```python
from build123d import *

# Parameters (mm, degrees)
F0_R            = 7.62
F1_DEPTH        = 25.4
F2_SIZE         = 2.54
F4_DEPTH        = 25.4
F4_COPIES_COUNT = 18
F6_R            = 5.08
F7_DEPTH        = 12.954
F8_R            = 5.08
F9_DEPTH        = 12.7


# Not quite as in the source:
# - a pattern or mirror of a feature is missing from the dataset's text; its kind, count and spacing are read off the source's solid


with BuildPart() as f1:
    # F0 (on Top) → F1 (new body)
    with BuildSketch(Plane.XY):
        Circle(F0_R)
    extrude(amount=F1_DEPTH)

    # F2
    f2_edges = [f1.edges().sort_by_distance(p)[0] for p in [
        (-7.62, 0, 25.4),
        (-7.62, 0, 0),
    ]]
    chamfer(f2_edges, length=F2_SIZE)

    # F3 (on face) → F4 (cut, through all)
    with BuildSketch(Plane.XY.offset(25.4)):
        with BuildLine():
            ThreePointArc((1.016, 7.5519629236), (0, 7.62), (-1.016, 7.5519629236))
            Line((-1.016, 7.5519629236), (-0.381, 5.588))
            Line((-0.381, 5.588), (0.381, 5.588))
            Line((0.381, 5.588), (1.016, 7.5519629236))
        make_face()
    f4 = extrude(amount=-F4_DEPTH, mode=Mode.SUBTRACT)

    # F4_copies: F4 ×18 about axis
    f4_copies_axis = Axis((0, 0, 0), (0, 0, 1))
    for i in range(1, F4_COPIES_COUNT):
        add(f4.rotate(f4_copies_axis, i * 360 / F4_COPIES_COUNT), mode=Mode.SUBTRACT)

    # F6 (on face) → F7 (join)
    with BuildSketch(Plane.XY.offset(25.4)):
        Circle(F6_R)
    extrude(amount=F7_DEPTH)

    # F8 (on face) → F9 (join)
    with BuildSketch(Plane(origin=(0, 0, 0), x_dir=(1, 0, 0), z_dir=(0, 0, -1))):
        Circle(F8_R)
    extrude(amount=F9_DEPTH)


solid = f1.part
```
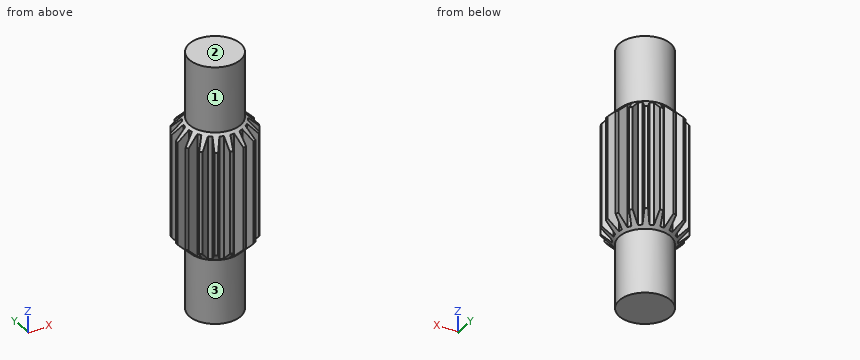
CAD build for the part. Positions are in the model's coordinates, mm. Face numbers are marked on the shaded views. A direction names the side the tool comes from. Coordinates: 2 decimals unless noted, no trailing zeros. Order: outer loops, then holes, each group sorted by start corner. A loop starts at its lowest first (then second) coordinate and runs counter-clockwise, first axis right, second up. Notation, with made-up numbers: (-16.75, -29) - (42.25, -29) arc R23 cw to (42.25, -11) - close; hole circle Ø8 at (83, -10). An arc over 180 degrees is marked (long way). Use a Markdown table: item, result. Add a question column.
(1) Drill centre lines: line 1 along Y through (x, z) = (6.5, 13); line 2 along Y through (x, z) = (-0.25, 21); line 3 along Y through (x, z) = (4.75, 18.5). Where is each one in solid material? Low to high. Write a range as [from, to].
(2) Saw through at A-A (z = 26). Give the cut face in (x, y).
(3) Which spindle directions (+Z, -Z, +X, -X, +Y, -Y) get a long thin tool onto all of the face, cutting with end or side? Do the marked faces 1, 2 and 3. Say none if no direction does.
(4) Flat gauge pins, fed straight in: pin 1 (2 mm diameter, centred on y = 0, z = 0.5, fed in from +X); pin 2 (8 mm diameter, centred on y = 4.5, z = 4.5, fed in from +X); pin 3 (8 mm diameter, centred on x = 6, z = -1, fed in from -Y). Where does each tip first touch, or does it go through?
Solved:
| question | item | result |
|---|---|---|
| 1 | line 1 | y = [-2.78, -1.91], [-0.47, 0.47], [1.91, 2.78] |
| 1 | line 2 | y = [-5.59, 5.59] |
| 1 | line 3 | y = [-4.58, -3.24], [-2.95, 2.95], [3.24, 4.58] |
| 2 | outline | circle Ø10.16 at (0, 0) |
| 3 | face 1 | +Z |
| 3 | face 2 | +Z, +X, -X, +Y, -Y |
| 3 | face 3 | -Z |
| 4 | pin 1 | stops at x = 6.58 |
| 4 | pin 2 | stops at x = 7.26 |
| 4 | pin 3 | stops at y = -6.4 |
